```python
from build123d import *

# Parameters (mm, degrees)
SKETCH1_W          = 10
SKETCH1_H          = 20
SKETCH2_R          = 5
CUT_EXTRUDE1_DEPTH = 20
CUT_EXTRUDE2_DEPTH = 10


with BuildPart() as part:
    # Sketch1 → Revolve1 (revolve)
    with BuildSketch(Plane.XY):
        with Locations((5, 10)):
            Rectangle(SKETCH1_W, SKETCH1_H)
    revolve(axis=Axis((0, 0, 0), (0, 1, 0)))

    # Sketch2 → Cut-Extrude1 (cut)
    with BuildSketch(Plane(origin=(0, 20, 0), x_dir=(1, 0, 0), z_dir=(0, 1, 0))):
        Circle(SKETCH2_R)
    extrude(amount=-CUT_EXTRUDE1_DEPTH, mode=Mode.SUBTRACT)

    # Sketch3 → Cut-Extrude2 (cut)
    with BuildSketch(Plane(origin=(0, 20, 0), x_dir=(1, 0, 0), z_dir=(0, 1, 0))):
        with BuildLine():
            Line((-10, 0), (-5, 0))
            ThreePointArc((-5, 0), (0, -5), (5, 0))
            Line((5, 0), (10, 0))
            ThreePointArc((10, 0), (0, -10), (-10, 0))
        make_face()
    extrude(amount=-CUT_EXTRUDE2_DEPTH, mode=Mode.SUBTRACT)


solid = part.part
```
Can you work these out from the model? Positions are in its coordinate system, mm. A direction names the side the tool comes from. Round coordinates to 2 decimals unless told otherwise and drop trailing zeros. Loops run counter-clockwise (first coordinate to the right, second up) from the corner with the lowest first, then second, coordinate; pieces in that order, holes last. Notation, with made-up numbers: (55, 9) -> (108, 9) arc R12 ccw to (108, 18) -> close; hole circle Ø3 at (-5.75, 3). An arc over 180 degrees is marked (long way). Answer in a Markdown table with one row per item.
Item 1: Suppose I cut it at B-B, the plane z = 1.5. List the corners of the cut face in (x, y) for me, plus the area to 3 significant figures.
Answer block:
| item | result |
|---|---|
| outline | (-9.89, 0) -> (-4.77, 0) -> (-4.77, 10) -> (-9.89, 10) -> close; (4.77, 0) -> (9.89, 0) -> (9.89, 10) -> (4.77, 10) -> close |
| area | 102 mm² |
Item 2: Will these pins go through, and if not, where does the flat tip stop? P1, Ø1.5, axis at x = -7.5, z = 5.5, coming from the +Y side; P2, Ø1.5, axis at x = -7.5, y = 2.5, coming from the -Z side; P3, Ø1.5, axis at x = 7.5, y = 14.5, coming from the +Z side; P4, Ø5, axis at x = 4.5, z = 7, coming from the -Y side.
Answer block:
| item | result |
|---|---|
| P1 | y = 10 |
| P2 | z = -7.38 |
| P3 | z = 0 |
| P4 | y = 0 |
Item 3: Suppose I cut it at D-D, the plane x = 7.5. List the corners of the cut face in (y, z) for me.
Answer block:
| item | result |
|---|---|
| outline | (0, -6.61) -> (20, -6.61) -> (20, 0) -> (10, 0) -> (10, 6.61) -> (0, 6.61) -> close |
Item 4: On a 3-axis mill with a long thin cutter (end or side, diameter ignored), from which of +Z, -Z, +X, -X, +Y, -Y can I reach the whole of each face in a straight line? I mean faces 4 (the flat face through (0, 20, -6)), 5 (the flat face through (0, 10, 6)). Say none if no direction works.
Answer block:
| item | result |
|---|---|
| face 4 | +Z, -Z, +X, -X, +Y |
| face 5 | +Z, +X, -X, +Y |
Item 5: We'd pull the mould along X, two halves only. Please class faces 1 (the flat face through (-8, 15, 0)), 2 (the cylindrical face through (-1.302, 7.918, -9.915)), 3 (the cylindrical face through (-0.651, 7.918, -4.957)): released by +X, released by -X, zero draft, split by the parting line, or undercut.
Answer block:
| item | result |
|---|---|
| face 1 | zero draft |
| face 2 | split by the parting line |
| face 3 | undercut |
Item 6: Suppose I cut it at A-A, the plane x = 0. List the corners of the cut face in (y, z) for me, plus the area to 3 significant figures.
Answer block:
| item | result |
|---|---|
| outline | (0, -10) -> (20, -10) -> (20, -5) -> (0, -5) -> close; (0, 5) -> (10, 5) -> (10, 10) -> (0, 10) -> close |
| area | 150 mm² |
Item 7: If I drill on probe 1 along X at (y, z) = (4.5, 0); probe 2 along Z at (x, y) = (-3.25, 4), over which ranges is the centre line in solid material (lowest first)?
Answer block:
| item | result |
|---|---|
| probe 1 | -10 to -5, 5 to 10 |
| probe 2 | -9.46 to -3.8, 3.8 to 9.46 |
Item 8: Suppose I cut it at C-C, the plane y = 9.5. List the corners of the cut face in (x, z) for me, plus the area to 3 significant figures.
Answer block:
| item | result |
|---|---|
| outline | circle Ø20 at (0, 0); hole circle Ø10 at (0, 0) |
| area | 236 mm² |
